Can you work these out from the drawing? Everything is in mm from the part's minimum corner. A direction names the side the tool comes from. Round coordinates to 2 decimals unless told otherwise and drop trailing zeros. Write each loop counter-clockwise with the first axis right and the second up, starting at its lowest first coordinate (ties: lowest second). Pieces come first, ordered by that corner, then holes. Notation, with made-up numbers: (-6, -4.75) -> (44, -4.75) arc R9 ccw to (44, 9.25) -> close; hole circle Ø5 at (5.5, -19.5). An arc over 180 degrees is marked (long way). Write item = value, one per line. Start each with the question number.
1) If I drill on line 1 (Z direction, x = 18, y = 19); line 2 (Y direction, x = 10.5, z = 3.25); line 3 (Y direction, x = 12.75, z = 18.25), over which ranges is the centre line in solid material (lowest first)?
2) For the marked faces 3, 4 and 5, which set-ups out of +Z, -Z, +X, -X, +Y, -Y let a thin tool reach every point of the face, with its end or its side?
3) Imagine slicing it at B-B, the plane z = 6.5. Please give me the cut outline in (x, y).
4) Thinking about a two-plate mould opening in Z: for the marked faces 1 and 2, which applies, +Z half, -Z half, draft (parallel to the pull), parting line (faces both ways), or undercut?
5) Imagine slicing it at A-A, the plane y = 10. Please give me the cut outline in (x, z), then the cut area to 3 significant figures.
6) I'm going to push flat-ended pins straight in: pin 1 (8 mm diameter, centred on y = 12, z = 3, fed in from -X); pin 2 (3.5 mm diameter, centred on x = 10, y = 10, fed in from +Z). Where does each tip first touch, or does it pass through?
7) Imagine slicing it at C-C, the plane z = 16.5. Please give me the cut outline in (x, y).
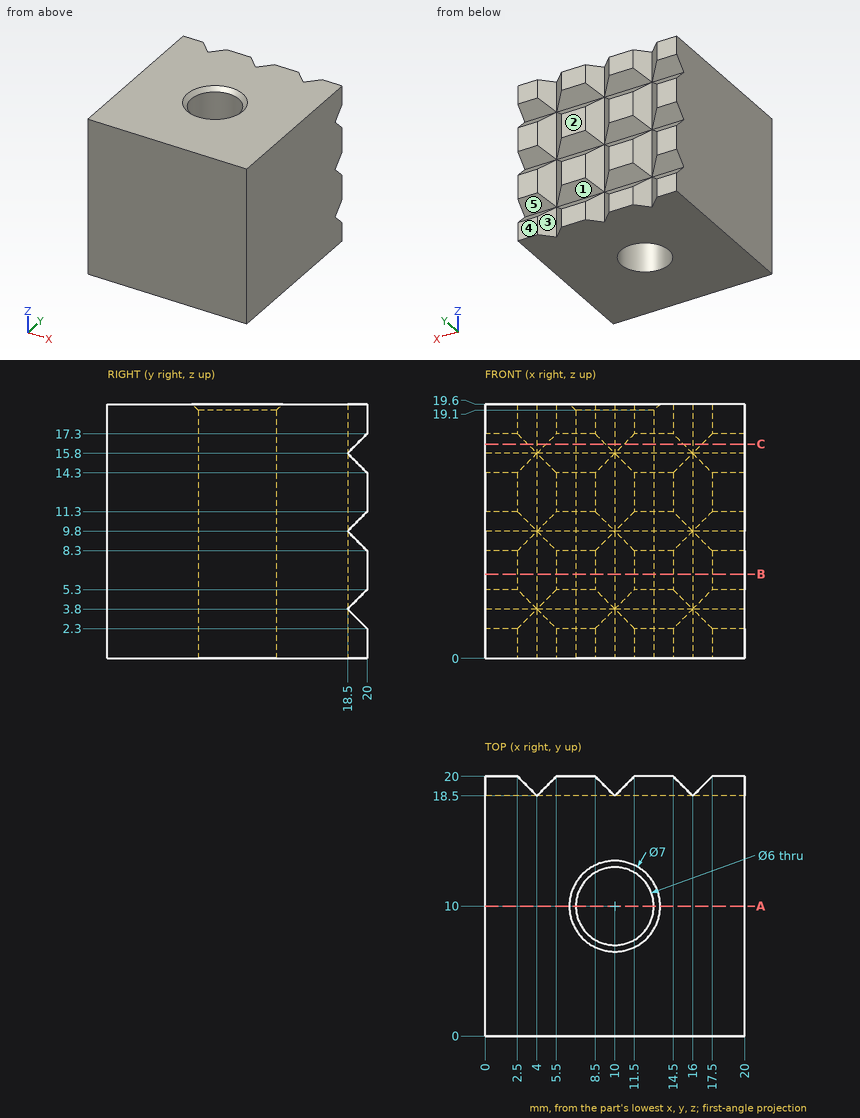
Reported:
q1.line_1 = 0 to 3.3, 4.3 to 9.3, 10.3 to 15.3, 16.3 to 19.6
q1.line_2 = 0 to 7.04, 12.96 to 19
q1.line_3 = 0 to 8.8, 11.2 to 20
q2.face_3 = +Z, -Z, +Y
q2.face_4 = +Z, -Z, +X, -X, +Y
q2.face_5 = +X, -X, +Y
q3.outline = (0, 0) -> (20, 0) -> (20, 20) -> (17.5, 20) -> (16, 18.5) -> (14.5, 20) -> (11.5, 20) -> (10, 18.5) -> (8.5, 20) -> (5.5, 20) -> (4, 18.5) -> (2.5, 20) -> (0, 20) -> close; hole circle Ø6 at (10, 10)
q4.face_1 = undercut
q4.face_2 = draft
q5.outline = (0, 0) -> (7, 0) -> (7, 19.1) -> (6.5, 19.6) -> (0, 19.6) -> close; (13, 0) -> (20, 0) -> (20, 19.6) -> (13.5, 19.6) -> (13, 19.1) -> close
q5.area = 274 mm²
q6.pin_1 = 0
q6.pin_2 = through
q7.outline = (0, 0) -> (20, 0) -> (20, 19.2) -> (16.7, 19.2) -> (16, 18.5) -> (15.3, 19.2) -> (10.7, 19.2) -> (10, 18.5) -> (9.3, 19.2) -> (4.7, 19.2) -> (4, 18.5) -> (3.3, 19.2) -> (0, 19.2) -> close; hole circle Ø6 at (10, 10)
